Autodesk Inventor part; units mm, degrees
ref_plane "YZ Plane" through (0, 0, 0) normal (1, 0, 0) x (0, 1, 0)
ref_plane "XZ Plane" through (0, 0, 0) normal (0, 1, 0) x (-1, 0, 0)
ref_plane "XY Plane" through (0, 0, 0) normal (0, 0, 1) x (1, 0, 0)
sketch "Sketch1" plane through (0, 0, 0) normal (0, 0, 1) x (1, 0, 0)
  line L0 (0, 0) -> (27, 0)
  line L1 (18, 17) -> (18, 20)
  line L2 (18, 20) -> (8, 20)
  line L3 (8, 20) -> (8, 17)
  line L4 (29, 17) -> (18, 17)
  line L5 (-3, 15) -> (-3, 5)
  line L6 (-3, 5) -> (0, 5)
  line L7 (0, 5) -> (0, 0)
  arc A0 (27, 0) -> (29, 2) centre (27, 2) ccw
  line L8 (-3, 15) -> (0, 15)
  line L9 (29, 17) -> (29, 2)
  line L10 (0, 15) -> (0, 17)
  line L11 (0, 17) -> (8, 17)
  point P0 (25, 0)
  dimension "d8" = 10
  dimension "d10" = 3
  dimension "d15" = 2
  dimension "d16" = 10
  dimension "d25" = 3
  dimension "d26" = 5
  dimension "d33" = 17
  dimension "d35" = 11
  dimension "d36" = 11
  dimension "d38" = 2
  dimension "d39" = 8
  dimension "d40" = 32
  dimension "d41" = 3
extrude "Extrusion1" add sketch "Sketch1" along normal blind 3
properties part number "OpenROV 2.3 Dev EChassis Horz Blinder"
Input: part model. Units: mm. Frame: model coordinates. A direction names the side the tool comes from. Coordinates: 2 decimals unless noted, no trailing zeros. Order: outer loops, then holes, each group sorted by start corner. A loop starts at its lowest first (then second) coordinate and runs counter-clockwise, first axis right, second up. Notation, with made-up numbers: (39.5, 40) - (57.5, 40) arc R25 ccw to (57.5, 79) - close; hole circle Ø9 at (54, 52.25). An arc over 180 degrees is marked (long way). Put each result on its own line as item: value.
1. Line query: line 1 along X through (y, z) = (3, 1.35); line 2 along Y through (x, z) = (-0.5, 2.4); line 3 along Y through (x, z) = (5.5, 1.3). Output: solid intervals per line, ascending.
Report:
line 1: x = 0 to 29
line 2: y = 5 to 15
line 3: y = 0 to 17
2. Reachability of faces 1 (the face through (24, 17, 1)), 2 (the face through (-2, 5, 1)), 3 (the face through (8, 19, 1)) from +Z, -Z, +X, -X, +Y, -Y: full face, straight path, thin tool, end or side. Return the list, or none.
Report:
face 1: +Z, -Z, +X, +Y
face 2: +Z, -Z, -X, -Y
face 3: +Z, -Z, -X, +Y
3. Cut plane A-A on z = 1.55. Return the cut outline in (x, y), then the cut area to 3 significant figures.
Report:
outline: (-3, 5) - (0, 5) - (0, 0) - (27, 0) arc R2 ccw to (29, 2) - (29, 17) - (18, 17) - (18, 20) - (8, 20) - (8, 17) - (0, 17) - (0, 15) - (-3, 15) - close
area: 552 mm2
4. Cut plane C-C on x = 1.5. Return the cut outline in (y, z).
Report:
outline: (0, 0) - (17, 0) - (17, 3) - (0, 3) - close
5. Contact query for flat-ended pins moving along their axis: pin 1 Ø1.5 at (x, z) = (-1.5, 1.5) entering from -Y; pin 2 Ø1.6 at (y, z) = (16.5, 2) entering from -X. Output: stop coordinate, or through.
Report:
pin 1: stops at y = 5
pin 2: stops at x = 0
6. Cut plane B-B on y = 17.5. Return the cut outline in (x, z).
Report:
outline: (8, 0) - (18, 0) - (18, 3) - (8, 3) - close
